Autodesk Inventor part; units mm, degrees
ref_plane "YZ Plane" through (0, 0, 0) normal (1, 0, 0) x (0, 1, 0)
ref_plane "XZ Plane" through (0, 0, 0) normal (0, 1, 0) x (-1, 0, 0)
ref_plane "XY Plane" through (0, 0, 0) normal (0, 0, 1) x (1, 0, 0)
sketch "Эскиз1" plane through (0, 0, 0) normal (0, 0, 1) x (1, 0, 0)
  circle A0 centre (82.5, -44) radius 1.5
  circle A1 centre (82.5, -114) radius 1.5
  circle A2 centre (81.5042, -129.3151) radius 1.5
  circle A3 centre (71.168, -167.8906) radius 1.5
  line L0 (82.5, -44) -> (82.5, -114) construction
  line L1 (81, -44) -> (81, -114)
  line L2 (84, -114) -> (84, -44)
  arc A4 (84, -44) -> (81, -44) centre (82.5, -44) ccw
  arc A5 (81, -114) -> (84, -114) centre (82.5, -114) ccw
  line L3 (82.5, -114) -> (81.5042, -129.3151) construction
  line L4 (81.0032, -113.9027) -> (80.0074, -129.2178)
  line L5 (83.001, -129.4125) -> (83.9968, -114.0973)
  arc A6 (83.9968, -114.0973) -> (81.0032, -113.9027) centre (82.5, -114) ccw
  arc A7 (80.0074, -129.2178) -> (83.001, -129.4125) centre (81.5042, -129.3151) ccw
  line L6 (81.5042, -129.3151) -> (71.168, -167.8906) construction
  line L7 (80.0553, -128.9269) -> (69.7191, -167.5023)
  line L8 (72.6168, -168.2788) -> (82.9531, -129.7034)
  arc A8 (82.9531, -129.7034) -> (80.0553, -128.9269) centre (81.5042, -129.3151) ccw
  arc A9 (69.7191, -167.5023) -> (72.6168, -168.2788) centre (71.168, -167.8906) ccw
  line L9 (82.5, -44) -> (71.168, -167.8906) construction
  line L10 (81.0062, -43.8634) -> (69.6742, -167.7539)
  line L11 (72.6617, -168.0272) -> (83.9938, -44.1366)
  arc A10 (83.9938, -44.1366) -> (81.0062, -43.8634) centre (82.5, -44) ccw
  arc A11 (69.6742, -167.7539) -> (72.6617, -168.0272) centre (71.168, -167.8906) ccw
  circle A12 centre (82.5, -44) radius 4
  circle A13 centre (82.5, -114) radius 4
  circle A14 centre (81.5042, -129.3151) radius 4
  circle A15 centre (71.168, -167.8906) radius 4
  point P0 (0, 0)
  point P1 (82.5, -79)
  point P2 (82.0021, -121.6576)
  point P3 (76.3361, -148.6029)
  point P4 (76.834, -105.9453)
  point P5 (84, -47.7081)
  point P6 (80.6685, -47.5561)
  point P7 (70.0119, -164.0613)
  point P8 (73.5766, -164.697)
  point P9 (81.9934, -133.2851)
  point P10 (83.2416, -125.7122)
  point P11 (83.7562, -117.7976)
  point P12 (84, -110.2919)
  dimension "d0" = 1.5
  dimension "d1" = 8
  dimension "d2" = 8
  dimension "d3" = 8
  dimension "d4" = 8
extrude "Выдавливание1" add sketch "Эскиз1" along normal blind 10 contours L2 A12 L11 A0 | A0 L10 A12 L2 | A0 L1 A12 L10 | L11 A12 L1 A0 | L2 A13 L1 L11 A12 | A12 L1 L11 L7 A15 L10 | L11 L1 A12 | A13 L5 A1 L2 | L2 A1 L1 A13 | A15 L7 A3 L10 | L10 A3 L8 A15 | L1 A13 L4 A14 L7 L11 | L1 L4 A13 | A15 L11 A3 L7 | L7 L11 A15 | L7 A14 L8 A15 L11 | L5 A13 L4 A1 | L5 A14 L4 A13 | A3 L11 A15 L8 | A14 L4 L7 | L7 L4 A2 L8 A14 | A14 L8 A2 L5 | L5 A2 L7 L4 A14 | L7 A2 L4
chamfer "Фаска1" distance 1 angle 45 8 edges at (81, -44, 10) (81, -114, 10) (80.0042, -129.3151, 10) (69.668, -167.8906, 10) (80.0042, -129.3151, 0) (81, -114, 0) (81, -44, 0) (69.668, -167.8906, 0)
properties part number "Шаблон2"
Part model, mm, in its own coordinate system. A direction names the side the tool comes from. Round coordinates to 2 decimals unless told otherwise and drop trailing zeros. Write each loop counter-clockwise with the first axis right and the second up, starting at its lowest first coordinate (ties: lowest second). Pieces come first, ordered by that corner, then holes.
Item 1: Cut at C-C, the plane x = 76.5. Give the cut face in (y, z).
Results:
outline: (-153.79, 0) - (-93.13, 0) - (-93.13, 10) - (-153.79, 10) - close
Item 2: Drop flat-ended pins along their axis: pin 1 Ø4 at (y, z) = (-64.5, 8) entering from -X; pin 2 Ø4 at (y, z) = (-91, 3) entering from +X; pin 3 Ø6 at (y, z) = (-119, 4.5) entering from -X; pin 4 Ø2.5 at (x, y) = (82.5, -114) entering from +Z. Give the stop position or say it passes through.
Results:
pin 1: stops at x = 78.94
pin 2: stops at x = 84
pin 3: stops at x = 73.86
pin 4: passes through
Item 3: Which spindle directions (+Z, -Z, +X, -X, +Y, -Y) get a long thin tool onto all of the face, cutting with end or side? Do faces 4 (the cylindrical face through (82.89, -128.74, 4.94)), 5 (the flat face through (75.415, -104.993, 4.93)), 6 (the flat face through (84, -79, 5)). Say none if no direction does.
Results:
face 4: +Z, -Z
face 5: +Z, -Z, -X
face 6: +Z, -Z, +X
Item 4: Two-plate mould, pull along X, no slides. Class faces 1 (the flat face through (77, -106, 10)), 2 (the flat face through (83.495, -121.81, 4.93)), 3 (the cylindrical face through (69.67, -167.96, 4.94)): +X half, -X half, draft (parallel to the pull), parting line (faces both ways), or undercut.
Results:
face 1: draft
face 2: +X half
face 3: undercut
Item 5: Cut at B-B, the plane z = 3. Give the cut face in (x, y), plus the area to 3 significant figures.
Results:
outline: (70.01, -164.06) arc R4 ccw (long way) to (73.58, -164.7) - (81.99, -133.29) arc R4 ccw to (83.24, -125.71) - (83.76, -117.8) arc R4 ccw to (84, -110.29) - (84, -47.71) arc R4 ccw (long way) to (80.67, -47.56) - close; hole circle Ø3 at (71.17, -167.89); hole circle Ø3 at (81.5, -129.32); hole (81, -114) arc R1.5 ccw (long way) to (81, -113.9) - (81, -113.95) - close; hole circle Ø3 at (82.5, -44)
area: 907 mm2
Item 6: Cut at D-D, the plane y = -74. Give the cut face in (x, z), plus the area to 3 significant figures.
Results:
outline: (78.25, 0) - (84, 0) - (84, 10) - (78.25, 10) - close
area: 57.5 mm2
Item 7: Cut at A-A, the plane y = -44. Give the cut face in (x, z), plus the area to 3 significant figures.
Results:
outline: (78.5, 0) - (80, 0) - (81, 1) - (81, 9) - (80, 10) - (78.5, 10) - close; (84, 1) - (85, 0) - (86.5, 0) - (86.5, 10) - (85, 10) - (84, 9) - close
area: 48.0 mm2
Item 8: Probe L1, parallel to Y at x = 84.75, z = 7; L2, parallel to X at y = -44, z = 7; L3, parallel to Y at x = 82.5, z = 5. List the from-to ranges inside material, lowest first.
Results:
L1: y = -131.65 to -126.98, -117.31 to -110.69, -47.31 to -40.69
L2: x = 78.5 to 81, 84 to 86.5
L3: y = -133.19 to -130.44, -128.19 to -115.5, -112.5 to -45.5, -42.5 to -40
